Build history of the part. All positions in model axes, mm. A direction names the side the tool comes from. Coordinates: 2 decimals unless noted, no trailing zeros. Loops run counter-clockwise (first coordinate to the right, second up) from the corner with the lowest first, then second, coordinate; pieces in that order, holes last. Notation, with made-up numbers: (12.25, 87) - (36.25, 87) arc R16 ccw to (36.25, 109) - close; hole circle Ø7 at (-31, 45.25). An arc over 180 degrees is marked (long way). One line per item, written item: value.
Autodesk Inventor part; units mm, degrees
ref_plane "YZ Plane" through (0, 0, 0) normal (1, 0, 0) x (0, 1, 0)
ref_plane "XZ Plane" through (0, 0, 0) normal (0, 1, 0) x (-1, 0, 0)
ref_plane "XY Plane" through (0, 0, 0) normal (0, 0, 1) x (1, 0, 0)
sketch "Skizze1" plane through (0, 0, 0) normal (0, 1, 0) x (-1, 0, 0)
  line L0 (6.8592, -116.2444) -> (0.8592, -116.2444)
  line L1 (0.8592, -116.2444) -> (0.8592, -56.2444)
  line L2 (6.8592, -56.2444) -> (6.8592, -116.2444)
  line L3 (7.8592, -116.2444) -> (-0.1408, -116.2444)
  line L4 (-0.1408, -116.2444) -> (-0.1408, -106.2444)
  line L5 (-0.1408, -106.2444) -> (7.8592, -106.2444)
  line L6 (7.8592, -106.2444) -> (7.8592, -116.2444)
  line L7 (3.8592, 157.3916) -> (3.8592, -262.6084)
  line L8 (6.8592, -56.2444) -> (0.8592, -56.2444)
  line L9 (0.8592, -56.2444) -> (-2.1408, -56.2444)
  line L10 (-2.1408, -56.2444) -> (-2.1408, -66.2444)
  line L11 (-2.1408, -66.2444) -> (0.8592, -66.2444)
  line L12 (0.8592, -66.2444) -> (0.8592, -56.2444)
  line L13 (6.8592, -56.2444) -> (9.8592, -56.2444)
  line L14 (9.8592, -56.2444) -> (9.8592, -66.2444)
  line L15 (9.8592, -66.2444) -> (6.8592, -66.2444)
  line L16 (6.8592, -66.2444) -> (6.8592, -56.2444)
  point P0 (0, 0)
  point P1 (0.8592, -106.2444)
  point P2 (6.8592, -106.2444)
  point P3 (6.8592, -116.2444)
  point P4 (3.8592, -116.2444)
  point P5 (6.8592, -66.2444)
  point P6 (0.8592, -66.2444)
  dimension "d1" = 60
  dimension "d9" = 6
  dimension "d25" = 8
  dimension "d26" = 10
  dimension "d27" = 1
  dimension "d44" = 3
  dimension "d45" = 10
  dimension "d46" = 3
extrude "Extrusion1" add sketch "Skizze1" along normal blind 3
sketch "Skizze2" plane through (0, 3, 0) normal (0, 1, 0) x (1, 0, 0)
  line L0 (-3.8592, 111.2444) -> (-6.8592, 111.2444) construction
  line L1 (-3.8592, 111.2444) -> (-0.8592, 111.2444) construction
  line L2 (-0.8592, 66.2444) -> (-0.8592, 106.2444) construction
  line L3 (-6.8592, 106.2444) -> (-6.8592, 66.2444) construction
  line L4 (0.1408, 116.2444) -> (-7.8592, 116.2444)
  point P0 (0, 0)
  point P1 (-0.8592, 56.2444)
  point P2 (-6.8592, 56.2444)
  point P3 (-0.8592, 16.2444)
  point P4 (-6.8592, 16.2444)
  dimension "d28" = 5
hole "Bohrung1" at (-3.8592, 3, -111.2444) direction (0, -1, 0) diameter 2.459 end through all
sketch "Skizze3" plane through (0.1408, 0, -116.2444) normal (0, 0, -1) x (-1, 0, 0)
  line L0 (4, 0) -> (4, 2.3)
  circle A0 centre (4, 2.3) radius 1.5
  line L1 (0, 0) -> (8, 0)
  point P0 (0.1408, 0)
  dimension "d29" = 3
  dimension "d30" = 2.3
extrude "Extrusion2" add sketch "Skizze3" along normal blind 3
sketch "Skizze5" plane through (0, 3, 0) normal (0, 1, 0) x (1, 0, 0)
  line L0 (2.1408, 56.2444) -> (-9.8592, 56.2444)
  line L1 (-9.8592, 66.2444) -> (2.1408, 66.2444)
  line L2 (2.1408, 66.2444) -> (2.1408, 56.2444)
  line L3 (-5.3592, 56.2444) -> (-2.3592, 56.2444)
  line L4 (-2.3592, 56.2444) -> (-2.3592, 66.2444)
  line L5 (-2.3592, 66.2444) -> (-5.3592, 66.2444)
  line L6 (-5.3592, 66.2444) -> (-5.3592, 56.2444)
  line L7 (-5.3592, 61.2444) -> (-9.8592, 61.2444) construction
  line L8 (-2.3592, 61.2444) -> (2.1408, 61.2444) construction
  line L9 (-9.8592, 66.2444) -> (-9.8592, 56.2444)
  point P0 (0, 0)
  point P1 (-2.3592, 56.2444)
  dimension "d43" = 3
extrude "Extrusion4" add sketch "Skizze5" along normal blind 20 contours L0 L4 L1 L2 | L0 L9 L1 L6
properties part number "SchubstangeA" material "PC/ABS-Kunststoff, 3DDruck, PLA"
Item 1: Cut at A-A, the plane y = 7.75. Write the cut outline in (x, z), then the cut area to 3 significant figures.
Check result:
outline: (-9.86, -66.24) - (-5.36, -66.24) - (-5.36, -56.24) - (-9.86, -56.24) - close; (-2.36, -66.24) - (2.14, -66.24) - (2.14, -56.24) - (-2.36, -56.24) - close
area: 90.0 mm^2
Item 2: Cut at C-C, the plane x = -4.5. Write the cut outline in (y, z), then the cut area to 3 significant figures.
Check result:
outline: (0, -116.24) - (0.94, -116.24) - (0.94, -119.24) - (3.66, -119.24) - (3.66, -116.24) - (3, -116.24) - (3, -112.29) - (0, -112.29) - close; (0, -110.2) - (3, -110.2) - (3, -56.24) - (0, -56.24) - close
area: 182 mm^2
Item 3: Cut at B-B, the plane z = -62. Write the cut outline in (x, y), then the cut area to 3 significant figures.
Check result:
outline: (-9.86, 0) - (2.14, 0) - (2.14, 23) - (-2.36, 23) - (-2.36, 3) - (-5.36, 3) - (-5.36, 23) - (-9.86, 23) - close
area: 216 mm^2
Item 4: Tool access for faces 1 (the face through (-2.75, 1.29, -117.72)), 2 (the face through (-0.859, 1, -87)), 3 (the face through (-5.359, 13, -61)), 4 (the face through (0, 23, -61)), 5 (the face through (0.141, 1, -111)): list every direction of +Z, -Z, +X, -X, +Y, -Y with a clear straight run to the whole face (end or side of a thin tool).
Check result:
face 1: -Z
face 2: +X, +Y, -Y
face 3: +Z, -Z, +Y
face 4: +Z, -Z, +X, -X, +Y
face 5: -Z, +X, +Y, -Y
Item 5: Drop flat-ended pins along their axis: P1, Ø5, axis at x = -1.5, y = 17, coming from the -Z side; P2, Ø1.5, axis at y = 1, z = -84, coming from the +X side; P3, Ø1.5, axis at y = 1, z = -109.5, coming from the -X side. Give the stop position or say it passes through.
Check result:
P1: stops at z = -66.24
P2: stops at x = -0.86
P3: stops at x = -7.86
Item 6: Pull direction Z, two halves, no side cores. Call faces 6 (the face through (-7, 11, -56.244)), 7 (the face through (-4, 2, -119.244)), 8 (the face through (-6.859, 1, -86)), 9 (the face through (-4, 0, -86)): released by +Z, released by -Z, zero draft, split by the parting line, or undercut.
Check result:
face 6: released by +Z
face 7: released by -Z
face 8: undercut
face 9: zero draft
Item 7: Cut at D-D, the plane y = 2.3. Write the cut outline in (x, z).
Check result:
outline: (-9.86, -66.24) - (-6.86, -66.24) - (-6.86, -106.24) - (-7.86, -106.24) - (-7.86, -116.24) - (-5.36, -116.24) - (-5.36, -119.24) - (-2.36, -119.24) - (-2.36, -116.24) - (0.14, -116.24) - (0.14, -106.24) - (-0.86, -106.24) - (-0.86, -66.24) - (2.14, -66.24) - (2.14, -56.24) - (-9.86, -56.24) - close; hole circle Ø2.46 at (-3.86, -111.24)
Item 8: Probe probe 1 along Z at (x, y) = (-7.25, 11.75); probe 2 along Y at (x, z) = (-5.5, -83.5); probe 3 along Z at (x, y) = (-1.75, 1.75). List the from-to ranges inside material, lowest first. Write a range as from..to.
Check result:
probe 1: z = -66.24..-56.24
probe 2: y = 0..3
probe 3: z = -116.24..-56.24
